```python
from build123d import *

# Parameters (mm, degrees)
F1_DEPTH = 1
F2_W     = 4
F2_H     = 4
F3_DEPTH = 41
F4_W     = 120
F4_H     = 2
F4_W_2   = 32
F4_W_3   = 56
F5_DEPTH = 4


with BuildPart() as f1:
    # F0 (on Top) → F1 (new body)
    with BuildSketch(Plane.XY):
        Polygon((0, 42), (0, 0), (24, 0), (24, 12), (120, 12), (120, 42), align=None)
    extrude(amount=F1_DEPTH)

    # F2 (on face) → F3 (join)
    with BuildSketch(Plane(origin=(0, 0, 0), x_dir=(1, 0, 0), z_dir=(0, 0, -1))):
        with Locations((22, -2)):
            Rectangle(F2_W, F2_H)
        with Locations((58, -14)):
            Rectangle(F2_W, F2_H)
        with Locations((118, -14)):
            Rectangle(F2_W, F2_H)
    extrude(amount=F3_DEPTH)

    # F4 (on face) → F5 (join)
    with BuildSketch(Plane(origin=(0, 0, 0), x_dir=(1, 0, 0), z_dir=(0, 0, -1))):
        with Locations((60, -41)):
            Rectangle(F4_W, F4_H)
        with Locations((40, -13)):
            Rectangle(F4_W_2, F4_H)
        with Locations((88, -13)):
            Rectangle(F4_W_3, F4_H)
    extrude(amount=F5_DEPTH)


solid = f1.part
```
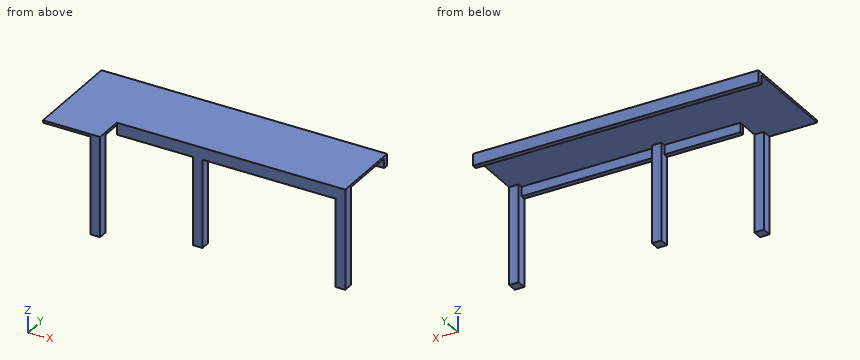
Design review of the part built by this model. Coordinates are the model's own, in mm. Give positions to 0.01 mm unless a question says otherwise; leave off trailing zeros. Order: outer loops, then holes, each group sorted by start corner. A loop starts at its lowest first (then second) coordinate and runs counter-clockwise, first axis right, second up. Notation, with made-up numbers: (58, -23.5) - (106, -23.5) arc R19 ccw to (106, -7.5) - close; hole circle Ø8 at (15.5, 78.25). An arc over 180 degrees is marked (long way). Use a Markdown table: item, result. Add a question column.
(1) Add section D-D on x = 9.5. Give the boundary of the cut face in (y, z).
(2) Add section B-B on x = 82.5. Give the boundary of the cut face in (y, z), then the cut area to 3 significant figures.
(3) Add section A-A on z = -31. Give the boundary of the cut face in (x, y), then the cut area to 3 significant figures.
(4) Clearance check with flat-ended pins moving along their axes: P1, Ø6, axis at x = 71, y = 28, coming from the -Z side; P2, Ø2, axis at x = 37.5, y = 13, coming from the -Z side; P3, Ø1.2, axis at y = 2.5, z = -13.5, coming from the -X side; P4, Ø12, axis at y = 17, z = -36.5, coming from the +X side. State where each tip first meets the part, or that it passes through.
(5) Add section C-C on y = 33.5. Give the boundary of the cut face in (x, z), then the cut area to 3 significant figures.
(6) Wall thickness on probe 1 along Z at (x, y) = (113, 16); probe 2 along Z at (x, y) = (97, 12.5): over which ranges is each line inside the solid? List them lowest first. Write a range as [from, to].
Report:
| question | item | result |
|---|---|---|
| 1 | outline | (0, 0) - (40, 0) - (40, -4) - (42, -4) - (42, 1) - (0, 1) - close |
| 2 | outline | (12, -4) - (14, -4) - (14, 0) - (40, 0) - (40, -4) - (42, -4) - (42, 1) - (12, 1) - close |
| 2 | area | 46.0 mm² |
| 3 | outline | (20, 0) - (24, 0) - (24, 4) - (20, 4) - close; (56, 12) - (60, 12) - (60, 16) - (56, 16) - close; (116, 12) - (120, 12) - (120, 16) - (116, 16) - close |
| 3 | area | 48.0 mm² |
| 4 | P1 | stops at z = 0 |
| 4 | P2 | stops at z = -4 |
| 4 | P3 | stops at x = 20 |
| 4 | P4 | stops at x = 120 |
| 5 | outline | (0, 0) - (120, 0) - (120, 1) - (0, 1) - close |
| 5 | area | 120 mm² |
| 6 | probe 1 | z = [0, 1] |
| 6 | probe 2 | z = [-4, 1] |
